```python
from build123d import *

# Parameters (mm, degrees)
SZKIC1_R                        = 12.7
DODANIE_WYCI_GNI_CIE1_DEPTH     = 0.054
SZKIC2_R                        = 6.35
DODANIE_WYCI_GNI_CIE2_DEPTH     = 6
WYTNIJ_WYCI_GNI_CIE1_DEPTH      = 19.953387982
WYTNIJ_WYCI_GNI_CIE1_DEPTH_BACK = 19.953387982
SZKIC3_R                        = 2.5
ZAOKR_GLENIE2_R                 = 1


with BuildPart() as part:
    # Szkic1 → Dodanie-wyciągnięcie1 (new body)
    with BuildSketch(Plane.XY):
        Circle(SZKIC1_R)
    extrude(amount=DODANIE_WYCI_GNI_CIE1_DEPTH)

    # Szkic2 → Dodanie-wyciągnięcie2 (add)
    with BuildSketch(Plane.XY.offset(0.054)):
        Circle(SZKIC2_R)
    extrude(amount=DODANIE_WYCI_GNI_CIE2_DEPTH)

    # Szkic3 → Wytnij-wyciągnięcie1 (cut, two sides: drawn at the far end of the back side and taken through both)
    with BuildSketch(Plane.XY.offset(6.054).offset(-WYTNIJ_WYCI_GNI_CIE1_DEPTH_BACK)):
        Circle(SZKIC3_R)
    extrude(amount=WYTNIJ_WYCI_GNI_CIE1_DEPTH + WYTNIJ_WYCI_GNI_CIE1_DEPTH_BACK, mode=Mode.SUBTRACT)

    # Zaokrąglenie2
    zaokr_glenie2_edges = [part.edges().sort_by_distance(p)[0] for p in [
        (-6.35, 0, 0.054),
        (-6.35, 0, 6.054),
    ]]
    fillet(zaokr_glenie2_edges, radius=ZAOKR_GLENIE2_R)


solid = part.part
```
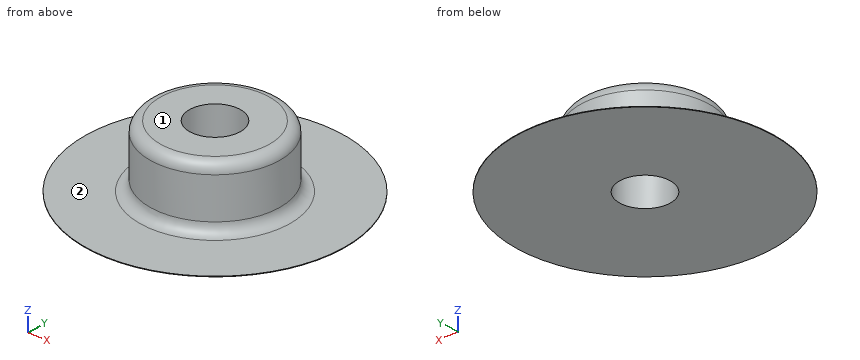
CAD build for the part. Positions are in the model's coordinates, mm. Face numbers are marked on the shaded views. A direction names the side the tool comes from. Round coordinates to 2 decimals unless told otherwise and drop trailing zeros. Order: outer loops, then holes, each group sorted by start corner. A loop starts at its lowest first (then second) coordinate and runs counter-clockwise, first axis right, second up. Notation, with made-up numbers: (82.25, -39) - (98.25, -39) arc R22 ccw to (98.25, -1) - close; hole circle Ø5 at (-36, -4.75). An arc over 180 degrees is marked (long way). Answer as CSV lines item,"result". Start each with the question number.
1. Tool access for the marked faces 1 and 2: list every direction of +Z, -Z, +X, -X, +Y, -Y with a clear straight run to the whole face (end or side of a thin tool).
2. Saw through at A-A, the plane y = 0. Write the cut outline in (x, z), and give its area (3 significant figures).
3. Saw through at C-C, the plane z = 4.5. Write the cut outline in (x, y).
4. Saw through at D-D, the plane y = 8.75. Write the cut outline in (x, z).
5. Pin check, flat tips, straight feed: pin 1 (3 mm diameter, centred on x = -6, z = 3, fed in from -Y); pin 2 (1 mm diameter, centred on y = 6, z = 1.5, fed in from -X); pin 3 (1.5 mm diameter, centred on x = 1.5, z = 5.5, fed in from +Y). Stop position of each tip, or through.
6. Drill centre lines: L1, parallel to Y at x = 0, z = 3; L2, parallel to X at y = 2.25, z = 4.25; L3, parallel to X at y = -1.5, z = 3. Where is each one in solid material? Low to high. Write a range as [from, to].
Model answer:
1,face 1,"+Z, +X, -X, +Y, -Y"
1,face 2,"+Z"
2,outline,"(-12.7, 0) - (-2.5, 0) - (-2.5, 6.05) - (-5.35, 6.05) arc R1 ccw to (-6.35, 5.05) - (-6.35, 1.05) arc R1 cw to (-7.35, 0.05) - (-12.7, 0.05) - close; (2.5, 0) - (12.7, 0) - (12.7, 0.05) - (7.35, 0.05) arc R1 cw to (6.35, 1.05) - (6.35, 5.05) arc R1 ccw to (5.35, 6.05) - (2.5, 6.05) - close"
2,area,"47.3 mm²"
3,outline,"circle Ø12.7 at (0, 0); hole circle Ø5 at (0, 0)"
4,outline,"(-9.2, 0) - (9.2, 0) - (9.2, 0.05) - (-9.2, 0.05) - close"
5,pin 1,"stops at y = -4.48"
5,pin 2,"stops at x = -3.17"
5,pin 3,"stops at y = 6.29"
6,L1,"y = [-6.35, -2.5], [2.5, 6.35]"
6,L2,"x = [-5.94, -1.09], [1.09, 5.94]"
6,L3,"x = [-6.17, -2], [2, 6.17]"
